Check sheet for the drawn part. Datum: minimum x, y, z corner. Units: mm. Round coordinates to 2 decimals unless told otherwise and drop trailing zeros. Order: outer loops, then holes, each group sorted by start corner. A loop starts at its lowest first (then second) coordinate and runs counter-clockwise, first axis right, second up. Notation, with made-up numbers: (-18, -26.5) -> (35, -26.5) arc R32 cw to (35, 9.5) -> close; hole circle Ø3 at (45, 88). An arc over 180 degrees is marked (long way). Answer in a Markdown table with one row per item.
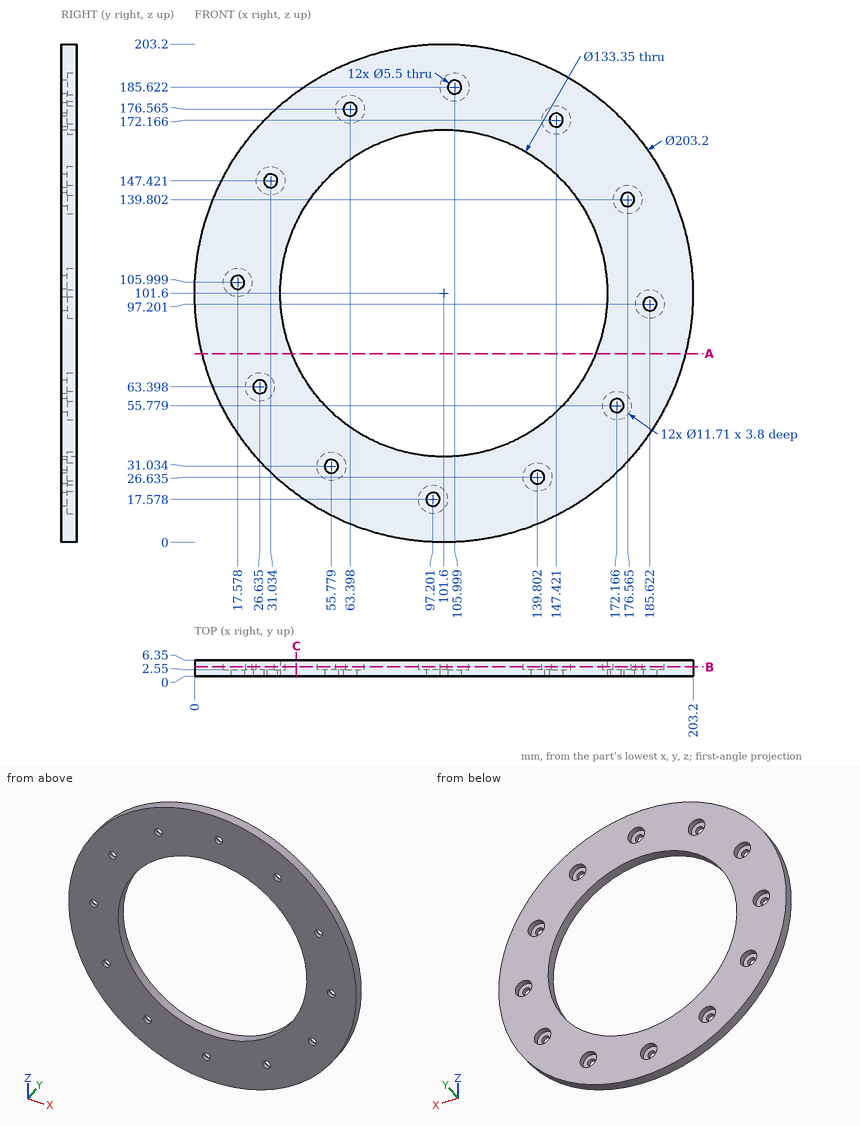
(1) Section check B-B on y = 3.75. Give the number of separate pieces and of enclosed holes in the cut face, plus the area to 3 significant figures.
Solutions:
| item | result |
|---|---|
| separate pieces | 1 |
| enclosed holes | 13 |
| area | 17,200 mm^2 |
(2) Scan lines: probe 1 along X at (y, z) = (0.75, 62.5) (1 decimal); probe 2 along Z at (x, y) = (65, 3.5) (1 decimal); probe 3 along Z at (x, y) = (116.5, 1.5). Record each from-to range of solid material in increasing order. Write a range as from..to.
Solutions:
| item | result |
|---|---|
| probe 1 | 7.8..24, 29.2..47.6, 155.6..195.4 |
| probe 2 | 6.8..45.9, 157.3..170.9, 182.2..196.4 |
| probe 3 | 1.1..36.61, 166.59..202.1 |
(3) Section check A-A on z = 77. Record the boundary of the cut face in (x, y).
Solutions:
| item | result |
|---|---|
| outline | (3.02, 0) -> (39.63, 0) -> (39.63, 6.35) -> (3.02, 6.35) -> close; (163.57, 0) -> (200.18, 0) -> (200.18, 6.35) -> (163.57, 6.35) -> close |
(4) Section check C-C on x = 41.5. Record the boundary of the cut face in (y, z).
Solutions:
| item | result |
|---|---|
| outline | (0, 19.68) -> (6.35, 19.68) -> (6.35, 72.73) -> (0, 72.73) -> close; (0, 130.47) -> (6.35, 130.47) -> (6.35, 183.52) -> (0, 183.52) -> close |
(5) Depth check by flat-ended pin: pin 1 Ø5 at (x, z) = (147.42, 172.17) entering from +Y; pin 2 Ø3.5 at (x, z) = (171.5, 58) entering from +Y; pin 3 Ø2 at (y, z) = (5.5, 27.5) entering from -X; pin 4 Ø1.5 at (y, z) = (3.5, 38.5) entering from -X. Enter the tip coordinate at first touch or a pass-through.
Solutions:
| item | result |
|---|---|
| pin 1 | through |
| pin 2 | y = 2.55 |
| pin 3 | x = 31.04 |
| pin 4 | x = 21.38 |
